Work out the finished part from the listing and answer in its coordinate system (mm). A direction names the side the tool comes from. Round coordinates to 2 decimals unless told otherwise and drop trailing zeros. Write each loop counter-clockwise with the first axis right and the second up, starting at its lowest first coordinate (ties: lowest second). Pieces come first, ordered by that corner, then holes.
1. Determine the mould class of faces 1 (the face through (60.84, -24.176, -232.176)), 2 (the face through (59.16, 45.323, -97.296)), 3 (the face through (59.16, 20.391, -266.834)) for opening direction Z: pulls with the +Z half, pulls with the -Z half, needs draft (parallel to the pull), parting line crosses it, or undercut.
2. Flat-ended cylindrical pins translate along their axes: pin 1 Ø8 at (x, y) = (73, -6) entering from -Z; pin 2 Ø18.5 at (x, z) = (79, -12) entering from -Y; pin 3 Ø3 at (x, z) = (62.5, -40.5) entering from +Y. Find the tip coordinate at first contact, or state that the pin passes through.
3. Straight lines are drawn through the part: probe 1 along Y at (x, z) = (74.5, -148.5); probe 2 along Z at (x, y) = (45, -4.5); probe 3 along Z at (x, y) = (22.5, -16). For each, find the intervals that lie inside material, in ascending order.
4. Find section A-A (x = 68). Write down the section's boundary in (y, z), and give its area (3 significant figures).
5. Find section B-B (y = -18.5). Write down the section's boundary in (x, z), and give its area (3 significant figures).
6. Find section D-D (z = -249.5). Write down the section's boundary in (x, y).
7. A tool of negligible diameter and unlimited length cuts with its end or side. For faces 4 (the face through (59, 0, -268)), 5 (the face through (59, 40.219, -235)), 6 (the face through (59, 0, -133)), 7 (the face through (59, 0, -8)), from which of +Z, -Z, +X, -X, +Y, -Y can it reach the whole face along a straight path? Write none if from no direction.
8. Find section C-C (z = -128). Write down the section's boundary in (x, y).
Autodesk Inventor part; units mm, degrees
ref_plane "YZ Plane" through (0, 0, 0) normal (1, 0, 0) x (0, 1, 0)
ref_plane "XZ Plane" through (0, 0, 0) normal (0, 1, 0) x (-1, 0, 0)
ref_plane "XY Plane" through (0, 0, 0) normal (0, 0, 1) x (1, 0, 0)
sketch "Sketch1" plane through (0, 0, 0) normal (1, 0, 0) x (0, 1, 0)
  line L0 (0, 0) -> (0, -280)
  line L1 (0, 0) -> (28.1328, -9.1597)
  line L2 (28.1328, -9.1597) -> (36.7239, -83.6155)
  line L3 (36.7239, -83.6155) -> (54.1655, -111.3657)
  line L4 (54.1655, -111.3657) -> (54.1655, -206.8716)
  line L5 (54.1655, -206.8716) -> (40.2194, -215.637)
  line L6 (40.2194, -215.637) -> (40.2194, -254.0323)
  line L7 (40.2194, -254.0323) -> (0, -280)
  dimension "d0" = 280
  dimension "d2" = 0
extrude "Extrusion1" add sketch "Sketch1" along normal blind 120
sketch "Sketch2" plane through (120, 0, 0) normal (1, 0, 0) x (0, 0, -1)
  line L0 (0, 0) -> (280, 0)
  circle A0 centre (38.4586, 0) radius 21.4935
  circle A1 centre (232.7073, 0) radius 24.1819
extrude "Extrusion2" add sketch "Sketch2" against normal blind 120
properties part number "car110th"
Worked answers:
1. face 1: undercut
1. face 2: pulls with the +Z half
1. face 3: pulls with the -Z half
2. pin 1: stops at z = -256.81
2. pin 2: stops at y = -12.88
2. pin 3: stops at y = 31.92
3. probe 1: y = 0 to 54.17
3. probe 2: z = -256.47 to -208.95, -59.48 to -17.44
3. probe 3: z = -250.84 to -214.58, -52.81 to -24.11
4. outline: (0, -280) - (40.22, -254.03) - (40.22, -215.64) - (54.17, -206.87) - (54.17, -111.37) - (36.72, -83.62) - (28.13, -9.16) - (0, 0) - (0, -16.97) arc R21.49 ccw to (0, -59.95) - (0, -208.53) arc R24.18 ccw to (0, -256.89) - close
4. area: 13,100 mm2
5. outline: (0, -248.28) - (120, -248.28) - (120, -217.13) - (0, -217.13) - close; (0, -49.4) - (120, -49.4) - (120, -27.52) - (0, -27.52) - close
5. area: 6,360 mm2
6. outline: (0, -17.4) - (120, -17.4) - (120, 40.22) - (0, 40.22) - close
7. face 4: -Z, +X, -X, -Y
7. face 5: -Z, +X, -X, +Y
7. face 6: +X, -X, -Y
7. face 7: +Z, +X, -X, -Y
8. outline: (0, 0) - (120, 0) - (120, 54.17) - (0, 54.17) - close
